The figure shows three views and two pictorial views of one solid part (mm, origin at its lowest corner). Answer the questions. A direction names the side the tool comes from. Round coordinates to 2 decimals unless told otherwise and drop trailing zeros. Order: outer loops, then holes, each group sorted by start corner. A loop starts at its lowest first (then second) coordinate and runs counter-clockwise, first axis right, second up. Notation, with made-up numbers: (46, 24) - (79, 24) arc R19 ccw to (79, 34) - close; hole circle Ø10 at (0.5, -16.5). An arc over 180 degrees is marked (long way). Answer as a JSON object with one key per item and string values. Group by question number.
Q1. Given pin 1 Ø1.6 at (x, y) = (32.5, 37.5) entering from -Z; pin 2 Ø2.5 at (y, z) = (19.5, 2) entering from -X, each flat-ended and moving along its own axis, determine where each tip first touches the part or whether it passes through.
Q2. A cutting plane is placed at A-A on x = 8. Determine the outline of the cut face in (y, z), and give its area (3 significant figures).
Q3. A cutting plane is placed at D-D on y = 20. Determine the outline of the cut face in (x, z).
Q4. A cutting plane is placed at C-C on y = 37.5. Determine the outline of the cut face in (x, z), and give its area (3 significant figures).
Q5. Consider line 1 (X direction, y = 37.5, z = 2.25); line 2 (Y direction, x = 32.5, z = 2.8); line 3 (Y direction, x = 21, z = 3.2). Determine where each line is inside the solid, lowest interval first.
Q6. The mould has two halves that part along Y. Classify the marked faces 4, 5 and 6: pulls with the +Y half, pulls with the -Y half, needs draft (parallel to the pull), parting line crosses it, or undercut.
Q7. A tool of negligible diameter and unlimited length cuts with its end or side. For the marked faces 1, 2 and 3, from which of +Z, -Z, +X, -X, +Y, -Y can it reach the whole face along a straight path? Write none if from no direction.
Q8. A cutting plane is placed at B-B on z = 0.6. Determine the outline of the cut face in (x, y).
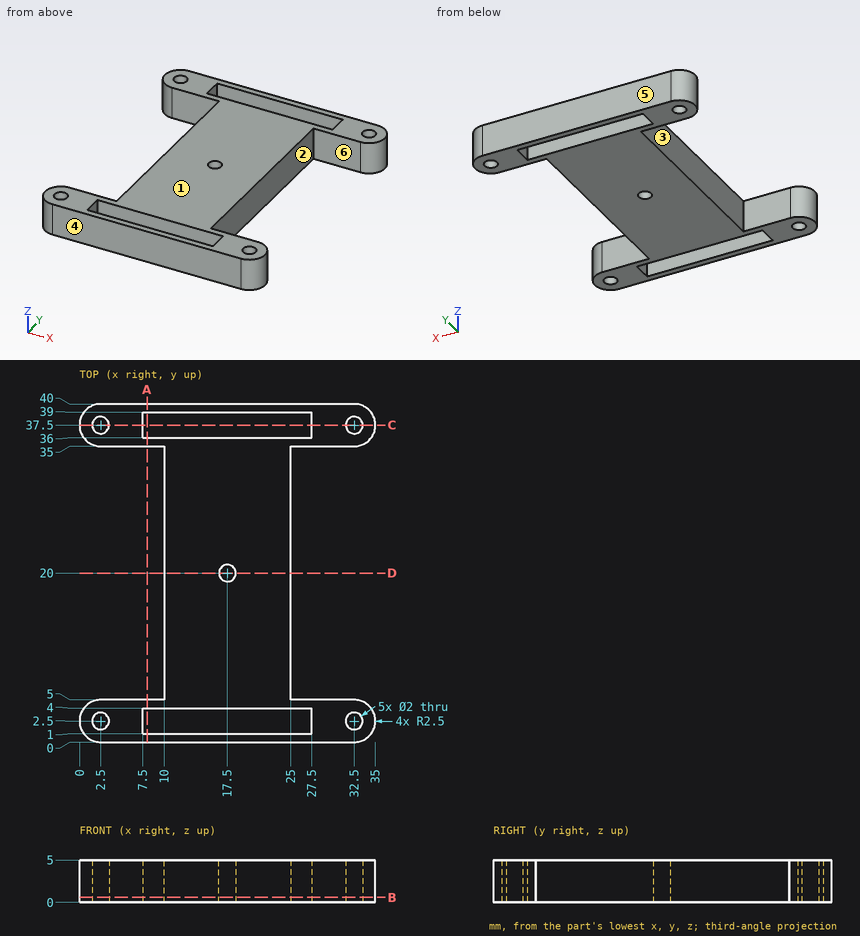
Result set:
{
 "1": {"pin 1": "passes through", "pin 2": "stops at x = 10"},
 "2": {"outline": "(0, 0) - (1, 0) - (1, 5) - (0, 5) - close; (4, 0) - (5, 0) - (5, 5) - (4, 5) - close; (35, 0) - (36, 0) - (36, 5) - (35, 5) - close; (39, 0) - (40, 0) - (40, 5) - (39, 5) - close", "area": "20.0 mm²"},
 "3": {"outline": "(10, 0) - (16.5, 0) - (16.5, 5) - (10, 5) - close; (18.5, 0) - (25, 0) - (25, 5) - (18.5, 5) - close"},
 "4": {"outline": "(0, 0) - (1.5, 0) - (1.5, 5) - (0, 5) - close; (3.5, 0) - (7.5, 0) - (7.5, 5) - (3.5, 5) - close; (27.5, 0) - (31.5, 0) - (31.5, 5) - (27.5, 5) - close; (33.5, 0) - (35, 0) - (35, 5) - (33.5, 5) - close", "area": "55.0 mm²"},
 "5": {"line 1": "x = 0 to 1.5, 3.5 to 7.5, 27.5 to 31.5, 33.5 to 35", "line 2": "y = 0 to 1.5, 3.5 to 5, 35 to 36.5, 38.5 to 40", "line 3": "y = 0 to 1, 4 to 36, 39 to 40"},
 "6": {"face 4": "pulls with the -Y half", "face 5": "pulls with the +Y half", "face 6": "undercut"},
 "7": {"face 1": "+Z, +X, -X, +Y, -Y", "face 2": "+Z, -Z, +X", "face 3": "+Z, -Z, -X"},
 "8": {"outline": "(2.5, 0) - (32.5, 0) arc R2.5 ccw to (32.5, 5) - (25, 5) - (25, 35) - (32.5, 35) arc R2.5 ccw to (32.5, 40) - (2.5, 40) arc R2.5 ccw to (2.5, 35) - (10, 35) - (10, 5) - (2.5, 5) arc R2.5 ccw to start; hole circle Ø2 at (2.5, 2.5); hole circle Ø2 at (2.5, 37.5); hole (7.5, 1) - (27.5, 1) - (27.5, 4) - (7.5, 4) - close; hole (7.5, 36) - (27.5, 36) - (27.5, 39) - (7.5, 39) - close; hole circle Ø2 at (17.5, 20); hole circle Ø2 at (32.5, 2.5); hole circle Ø2 at (32.5, 37.5)"}
}
